Source: CAD feature listing. Evaluate the final solid. Frame: model axes, mm. Face numbers are marked on the shaded views. A direction names the side the tool comes from. Give positions to 0.01 mm unless a question says otherwise; leave off trailing zeros. Loops run counter-clockwise (first coordinate to the right, second up) from the corner with the lowest first, then second, coordinate; pieces in that order, holes last. Notation, with made-up numbers: (13, -14) -> (56, -14) arc R26 ccw to (56, 4) -> close; hole circle Ø2 at (68, -33). An arc over 180 degrees is marked (long way). Return JSON: item names as keys, results as strings. Group by question number.
(1) Pin query (flat end, axial travel): pin 1 (1.5 mm diameter, centred on y = -17.5, z = 14, fed in from -X); pin 2 (3 mm diameter, centred on x = 56.5, z = -5, fed in from +Y); pin 3 (5 mm diameter, centred on x = 131.5, y = 2.5, fed in from -Z). Return the tip coordinate at first contact, or that it passes through.
(2) Access query for the marked faces 1, 2 and 3. Directions: +Z, -Z, +X, -X, +Y, -Y. A direction counts if a zero-diameter tool reaches every point of the face in a straight line with its end or side. Return the directions, or none.
(3) Ray query, line 1 (X direction, y = -12, z = 20.5); line 2 (Z direction, x = 166.5, y = 12); line 3 (Y direction, x = 104, z = 1). Return the intervals inside material, ascending. Write a range as from..to.
(4) Cut plane A-A on z = 0. Return loops of the section in (x, y).
(5) Cut plane C-C on x = 64. Return loops of the section in (y, z), then the cut area to 3 significant figures.
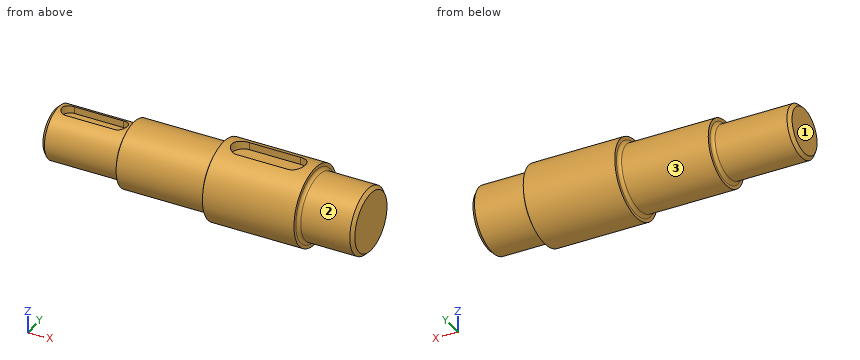
```python
from build123d import *

# Parameters (mm, degrees)
CHAMFER_1_SIZE      = 2
FILLET_1_R          = 2
CUT_EXTRUDE_1_DEPTH = 5
CUT_EXTRUDE_2_DEPTH = 5.5


with BuildPart() as part:
    # Эскиз1 → Повернуть1 (revolve)
    with BuildSketch(Plane.XY):
        Polygon((0, 0), (0, 16), (48, 16), (48, 20), (103, 20), (103, 24), (159, 24), (159, 20), (193, 20), (193, 0), align=None)
    revolve(axis=Axis((193, 0, 0), (-1, 0, 0)))

    # Фаска1
    chamfer_1_edges = [part.edges().sort_by_distance(p)[0] for p in [
        (0, -16, 0),
        (193, -20, 0),
    ]]
    chamfer(chamfer_1_edges, length=CHAMFER_1_SIZE)

    # Скругление1
    fillet_1_edges = [part.edges().sort_by_distance(p)[0] for p in [
        (48, -16, 0),
        (159, -20, 0),
        (103, -20, 0),
    ]]
    fillet(fillet_1_edges, radius=FILLET_1_R)

    # Эскиз2 → Вырез-Вытянуть1 (cut)
    with BuildSketch(Plane.XY.offset(16)):
        with BuildLine():
            Line((9, 5), (39, 5))
            ThreePointArc((39, 5), (44, 0), (39, -5))
            Line((39, -5), (9, -5))
            ThreePointArc((9, -5), (4, 0), (9, 5))
        make_face()
    extrude(amount=-CUT_EXTRUDE_1_DEPTH, mode=Mode.SUBTRACT)

    # Эскиз3 → Вырез-Вытянуть2 (cut)
    with BuildSketch(Plane.XY.offset(24)):
        with BuildLine():
            Line((115, 7), (146, 7))
            ThreePointArc((146, 7), (153, 0), (146, -7))
            Line((146, -7), (115, -7))
            ThreePointArc((115, -7), (108, 0), (115, 7))
        make_face()
    extrude(amount=-CUT_EXTRUDE_2_DEPTH, mode=Mode.SUBTRACT)


solid = part.part
```
Answers:
{
 "1": {"pin 1": "x = 102.97", "pin 2": "y = 19.69", "pin 3": "z = -24"},
 "2": {"face 1": "+Z, -Z, -X, +Y, -Y", "face 2": "+X", "face 3": "-X"},
 "3": {"line 1": "103..159", "line 2": "-16..16", "line 3": "-23.98..23.98"},
 "4": {"outline": "(0, -14) -> (2, -16) -> (46, -16) arc R2 cw to (48, -18) -> (48, -20) -> (101, -20) arc R2 cw to (103, -22) -> (103, -24) -> (159, -24) -> (159, -22) arc R2 cw to (161, -20) -> (191, -20) -> (193, -18) -> (193, 18) -> (191, 20) -> (161, 20) arc R2 cw to (159, 22) -> (159, 24) -> (103, 24) -> (103, 22) arc R2 cw to (101, 20) -> (48, 20) -> (48, 18) arc R2 cw to (46, 16) -> (2, 16) -> (0, 14) -> close"},
 "5": {"outline": "circle Ø40 at (0, 0)", "area": "1,260 mm²"}
}
